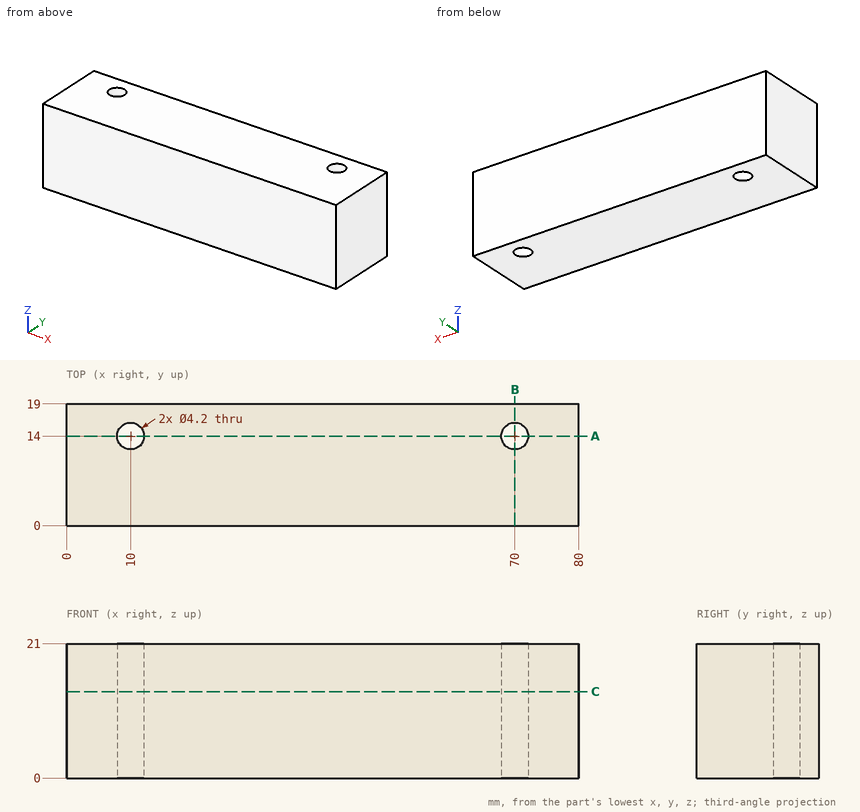
Verification items for this drawing (mm, ordinates from the low corner). Coordinates: 2 decimals unless noted, no trailing zeros. Order: outer loops, then holes, each group sorted by start corner. A loop starts at its lowest first (then second) coordinate and runs counter-clockwise, first axis right, second up. Notation, with made-up numbers: (-38, 47) - (16, 47) arc R21 ccw to (16, 78) - close; hole circle Ø5 at (80, 24.25). An arc over 180 degrees is marked (long way). Answer in a Markdown table with one row per item. Add a question column.
1. Gauge pin test, flat end, axial feed: pin 1 Ø3.5 at (x, y) = (10, 14) entering from -Z. Record the tip position at first contact, or that the pin passes through.
2. Section check A-A (y = 14). Enter the section's corners in (x, z).
3. Section check C-C (z = 13.5). Enter the section's corners in (x, y).
4. Section check B-B (x = 70). Enter the section's corners in (y, z).
5. Material ranges on L1, parallel to Y at x = 70, z = 9.5; L2, parallel to X at y = 14.25, z = 19.5; L3, parallel to X at y = 13, z = 18, recorded low to high. Write a range as [from, to].
Data:
| question | item | result |
|---|---|---|
| 1 | pin 1 | passes through |
| 2 | outline | (0, 0) - (7.9, 0) - (7.9, 21) - (0, 21) - close; (12.1, 0) - (67.9, 0) - (67.9, 21) - (12.1, 21) - close; (72.1, 0) - (80, 0) - (80, 21) - (72.1, 21) - close |
| 3 | outline | (0, 0) - (80, 0) - (80, 19) - (0, 19) - close; hole circle Ø4.2 at (10, 14); hole circle Ø4.2 at (70, 14) |
| 4 | outline | (0, 0) - (11.9, 0) - (11.9, 21) - (0, 21) - close; (16.1, 0) - (19, 0) - (19, 21) - (16.1, 21) - close |
| 5 | L1 | y = [0, 11.9], [16.1, 19] |
| 5 | L2 | x = [0, 7.91], [12.09, 67.91], [72.09, 80] |
| 5 | L3 | x = [0, 8.15], [11.85, 68.15], [71.85, 80] |
